from build123d import *

# Parameters (mm, degrees)
F3_DEPTH = 165
F4_SIZE  = 79.99999
F5_R     = 6
F6_DEPTH = 50
F7_W     = 116
F7_H     = 90
F8_DEPTH = 5
F9_R     = 10


# Not quite as in the source:
# - a fillet or chamfer is up to 0.001 mm smaller than in the source, because OpenCascade refuses the exact size


with BuildPart() as f3:
    # F2 (on Right) → F3 (new body, symmetric)
    with BuildSketch(Plane.YZ):
        Polygon((-40, 75), (-40, -75), (40, -75), (40, 15), (0, 15), (0, 75), align=None)
    extrude(amount=F3_DEPTH, both=True)

    # F4 (size 80 in the source; OpenCascade refuses exactly that, so slightly less here)
    f4_edges = [f3.edges().sort_by_distance(p)[0] for p in [
        (-165, 40, -30),
        (165, -40, 0),
    ]]
    chamfer(f4_edges, length=F4_SIZE)

    # F5 (on face) → F6 (cut)
    with BuildSketch(Plane(origin=(0, 40, 0), x_dir=(-1, 0, 0), z_dir=(0, 1, 0))):
        with Locations((35, -5)):
            Circle(F5_R)
        with Locations((55, -45)):
            Circle(F5_R)
        with Locations((-115, -5)):
            Circle(F5_R)
        with Locations((-135, -45)):
            Circle(F5_R)
    extrude(amount=-F6_DEPTH, mode=Mode.SUBTRACT)

    # F7 (on face) → F8 (cut)
    with BuildSketch(Plane(origin=(0, 40, 0), x_dir=(-1, 0, 0), z_dir=(0, 1, 0))):
        with Locations((67, -30)):
            Rectangle(F7_W, F7_H)
        with Locations((-147, -30)):
            Rectangle(F7_W, F7_H)
    extrude(amount=-F8_DEPTH, mode=Mode.SUBTRACT)

    # F9
    f9_edges = [f3.edges().sort_by_distance(p)[0] for p in [
        (-39.999995, -40, 75),
    ]]
    fillet(f9_edges, radius=F9_R)


solid = f3.part
Check sheet for the modelled part. Datum: model origin and axes. Units: mm. A direction names the side the tool comes from. Coordinates: 2 decimals unless noted, no trailing zeros. Write each loop counter-clockwise with the first axis right and the second up, starting at its lowest first coordinate (ties: lowest second). Pieces come first, ordered by that corner, then holes.
Item 1: Access from +Z, -Z, +X, -X, +Y, -Y to the whole of each face (thin tool, end or side, straight path). Record for faces 4 (the face through (125, 35, -29)), 5 (the face through (113, -10, -5)), 6 (the face through (2, 0, 45)), 7 (the face through (-49, 35, -29)), 8 (the face through (-35, -10, -5)).
Numbers:
face 4: +Z, -Z, +X, +Y
face 5: +X, +Y
face 6: +Z, +X, -X, +Y
face 7: +Z, -Z, -X, +Y
face 8: +Y
Item 2: Cross-section at B-B on x = 82. Record the boundary of the cut face in (y, z), then the cut area to 3 significant figures.
Numbers:
outline: (-40, -75) - (40, -75) - (40, 15) - (0, 15) - (0, 75) - (-30, 75) arc R10 ccw to (-40, 65) - close
area: 9,580 mm2
Item 3: Mould release check, pull along X, two halves, no side actions. Record for faces 1 (the face through (109.277, 12.815, -3.198)), 2 (the face through (19, 20, 15)), 3 (the face through (115, -10, -16)): released by +X, released by -X, zero draft, split by the parting line, or undercut.
Numbers:
face 1: undercut
face 2: zero draft
face 3: released by +X
Item 4: Scan lines: probe 1 along Z at (x, y) = (-35, 4); probe 2 along X at (y, z) = (5.5, -1); probe 3 along Y at (x, z) = (-13, -19). Record each from-to range of solid material in increasing order.
Numbers:
probe 1: z = -75 to -11, 1 to 15
probe 2: x = -119.5 to -39.47, -30.53 to 110.53, 119.47 to 130.5
probe 3: y = -40 to 35
Item 5: Depth check by flat-ended pin: pin 1 Ø3 at (x, z) = (-35, -8.5) entering from +Y; pin 2 Ø7 at (x, z) = (115, -5) entering from -Y; pin 3 Ø15.5 at (x, z) = (-55, -45) entering from +Y; pin 4 Ø5.5 at (y, z) = (36.5, -19) entering from +X. Enter the tip coordinate at first touch or a pass-through.
Numbers:
pin 1: stops at y = -10
pin 2: stops at y = -13.5
pin 3: stops at y = 35
pin 4: stops at x = 160
Item 6: Cross-section at C-C on y = 20. Record the boundary of the cut face in (x, z), then the cut area to 3 significant figures.
Numbers:
outline: (-105, -75) - (145, -75) - (145, 15) - (-105, 15) - close; hole circle Ø12 at (-55, -45); hole circle Ø12 at (-35, -5); hole circle Ø12 at (115, -5); hole circle Ø12 at (135, -45)
area: 22,000 mm2
